```python
from build123d import *

# Parameters (mm, degrees)
BOSS_EXTRUDE1_DEPTH     = 40
CUT_EXTRUDE1_DEPTH      = 8
CUT_EXTRUDE2_DEPTH      = 120.290091807
CUT_EXTRUDE2_DEPTH_BACK = 120.290091807
SKETCH3_R               = 15


with BuildPart() as part:
    # Sketch1 → Boss-Extrude1 (new body)
    with BuildSketch(Plane(origin=(0, 0, 0), x_dir=(1, 0, 0), z_dir=(0, 1, 0))):
        with BuildLine():
            Line((0, 0), (50, 0))
            Line((50, 0), (79.69848481, 29.69848481))
            ThreePointArc((79.69848481, 29.69848481), (82.04163056, 35.355339059), (79.69848481, 41.012193309))
            Line((79.69848481, 41.012193309), (46.246943589, 74.463734529))
            ThreePointArc((46.246943589, 74.463734529), (38.809068701, 76.606108799), (33.038444811, 71.447460693))
            ThreePointArc((33.038444811, 71.447460693), (20.256617737, 54.457585283), (0, 48))
            ThreePointArc((0, 48), (-14, 34), (0, 20))
            Line((0, 20), (0, 0))
        make_face()
    extrude(amount=BOSS_EXTRUDE1_DEPTH)

    # Sketch2 → Cut-Extrude1 (cut)
    with BuildSketch(Plane(origin=(0, 40, 0), x_dir=(1, 0, 0), z_dir=(0, 1, 0))):
        with BuildLine():
            Line((20, 10), (20, 40.573593129))
            ThreePointArc((20, 40.573593129), (17.886751346, 44.656076033), (13.333333333, 45.287638337))
            ThreePointArc((13.333333333, 45.287638337), (6.764079149, 43.576057614), (0, 43))
            ThreePointArc((0, 43), (-9, 34), (0, 25))
            ThreePointArc((0, 25), (3.535533906, 23.535533906), (5, 20))
            Line((5, 20), (5, 10))
            ThreePointArc((5, 10), (6.464466094, 6.464466094), (10, 5))
            Line((10, 5), (15, 5))
            ThreePointArc((15, 5), (18.535533906, 6.464466094), (20, 10))
        make_face()
    extrude(amount=-CUT_EXTRUDE1_DEPTH, mode=Mode.SUBTRACT)

    # Sketch3 → Cut-Extrude2 (cut, two sides: drawn at the far end of the back side and taken through both)
    with BuildSketch(Plane.XY.offset(-CUT_EXTRUDE2_DEPTH_BACK)):
        with Locations(Location((50, 20, 0), (0, 0, 90))):
            Circle(SKETCH3_R)
        with BuildLine():
            Line((-14, 28), (-14, 12))
            ThreePointArc((-14, 12), (-6, 20), (-14, 28))
        make_face()
    extrude(amount=CUT_EXTRUDE2_DEPTH + CUT_EXTRUDE2_DEPTH_BACK, mode=Mode.SUBTRACT)


solid = part.part
```
For this review, take the finished solid that the model builds, in its own axes (mm). A direction names the side the tool comes from. Round coordinates to 2 decimals unless told otherwise and drop trailing zeros. Write each loop counter-clockwise with the first axis right and the second up, starting at its lowest first coordinate (ties: lowest second). Pieces come first, ordered by that corner, then holes.
1) Machinability: for faces 4 (the face through (33, 0, -30)), 5 (the face through (9, 32, -26)), 6 (the face through (0, 20, -10)), which of the approach directions +Z, -Z, +X, -X, +Y, -Y give a long, thin tool a straight path to every point of the face, cutting with its end or side? Answer none if there is none.
Answer below:
face 4: +Z, -Z, +X, -X, -Y
face 5: +Y
face 6: +Z, -X, +Y, -Y
2) Take a section at D-D on y = 9.5. Give the boundary of the cut face in (x, z), then the cut area to 3 significant figures.
Answer below:
outline: (0, -48) arc R35 cw to (33.04, -71.45) arc R8 ccw to (39.29, -76.7) - (39.29, 0) - (0, 0) - (0, -20) arc R14 ccw to start; (60.71, -60) - (79.7, -41.01) arc R8 ccw to (79.7, -29.7) - (60.71, -10.71) - close
area: 3,170 mm2
3) Mouldability with a two-part tool opening along Z and no side actions: class faces 1 (the face through (66.92, 19.72, -53.79)), 2 (the face through (18, 36, -6)), 3 (the face through (35.128, 18.047, -38.943)) as +Z half, -Z half, draft (parallel to the pull), parting line (faces both ways), or undercut.
Answer below:
face 1: -Z half
face 2: undercut
face 3: draft
4) Take a section at C-C on x = 17. Give the boundary of the cut face in (y, z), then the cut area to 3 significant figures.
Answer below:
outline: (0, -52.41) - (40, -52.41) - (40, -45.16) - (32, -45.16) - (32, -5.42) - (40, -5.42) - (40, 0) - (0, 0) - close
area: 1,780 mm2
5) Take a section at B-B on y = 20. Give the boundary of the cut face in (x, z).
Answer below:
outline: (-6, -46.65) arc R14 ccw to (0, -48) arc R35 cw to (33.04, -71.45) arc R8 ccw to (35, -74.53) - (35, 0) - (0, 0) - (0, -20) arc R14 ccw to (-6, -21.35) - close; (65, -55.71) - (79.7, -41.01) arc R8 ccw to (79.7, -29.7) - (65, -15) - close
6) Insertion check: pin 1 Ø6.5 at (y, z) = (36.5, -28) entering from -X; pin 2 Ø10 at (y, z) = (18, -9.5) entering from -X; pin 3 Ø10 at (y, z) = (19.5, -57) entering from -X. Each pin has a flat end and moves straight along its axis. Give the tip position at first contact, or say it passes through.
Answer below:
pin 1: stops at x = -13.73
pin 2: stops at x = 0
pin 3: stops at x = 16.25
7) Take a section at A-A on z = -31.5. Give the boundary of the cut face in (x, y).
Answer below:
outline: (-13.77, 0) - (81.05, 0) - (81.05, 40) - (20, 40) - (20, 32) - (-8.65, 32) - (-8.65, 40) - (-13.77, 40) - (-13.77, 28) arc R8 cw to (-13.77, 12) - close; hole circle Ø30 at (50, 20)
8) For line 1 along Y through (x, z) = (50, -26); line 2 along X through (y, z) = (28, -22.5); line 3 along X through (y, z) = (37.5, -14), list the stretches that pass through material, from the lowest coordinate up.
Answer below:
line 1: y = 0 to 5, 35 to 40
line 2: x = -7.98 to 37.31, 62.69 to 72.5
line 3: x = 0 to 5, 20 to 64
